Source: CAD feature listing. Evaluate the final solid. Frame: model axes, mm. Round coordinates to 2 decimals unless told otherwise and drop trailing zeros. Loops run counter-clockwise (first coordinate to the right, second up) from the corner with the lowest first, then second, coordinate; pieces in that order, holes last.
Item 1: Section query A-A on z = 23.57. Return loops of the section in (x, y).
Item 2: Section query B-B on x = -42.12. Return loops of the section in (y, z), then the cut area to 3 significant figures.
Item 3: Section query D-D on x = -17.5. Return loops of the section in (y, z).
Item 4: Ray query, L1, parallel to X at y = 1.5, z = -23.57; L2, parallel to Z at x = 32, y = 2.1; L3, parallel to Z at x = -30.5, y = 0.7. Return the intervals inside material, ascending.
Item 5: Section query C-C on x = 32.5. Return loops of the section in (y, z).
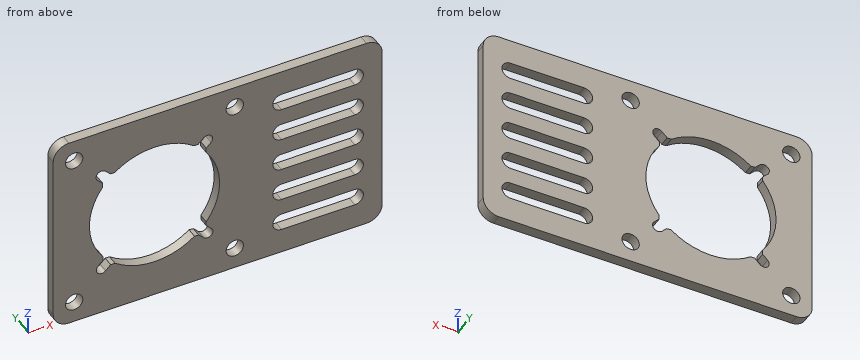
```python
from build123d import *

# Parameters (mm, degrees)
SKETCH1_W           = 96.5
SKETCH1_H           = 60
BOSS_EXTRUDE1_DEPTH = 3
SKETCH2_R           = 2.55
SKETCH2_W           = 26.6
SKETCH2_H           = 5.1
CUT_EXTRUDE1_DEPTH  = 57.895188725
FILLET1_R           = 2.55
FILLET2_R           = 4.6


with BuildPart() as part:
    # Sketch1 → Boss-Extrude1 (new body)
    with BuildSketch(Plane(origin=(0, 0, 0), x_dir=(1, 0, 0), z_dir=(0, 1, 0))):
        Rectangle(SKETCH1_W, SKETCH1_H)
    extrude(amount=BOSS_EXTRUDE1_DEPTH)

    # Sketch2 → Cut-Extrude1 (cut, through all)
    with BuildSketch(Plane(origin=(0, 3, 0), x_dir=(1, 0, 0), z_dir=(0, 1, 0))):
        with Locations(Location((-42.12, 23.57, 0), (0, 0, 270))):
            Circle(SKETCH2_R)
        with Locations(Location((5.02, 23.57, 0), (0, 0, 270))):
            Circle(SKETCH2_R)
        with Locations(Location((5.02, -23.57, 0), (0, 0, 270))):
            Circle(SKETCH2_R)
        with Locations(Location((-42.12, -23.57, 0), (0, 0, 270))):
            Circle(SKETCH2_R)
        with Locations((29.45, 20)):
            Rectangle(SKETCH2_W, SKETCH2_H)
        with Locations((29.45, 10)):
            Rectangle(SKETCH2_W, SKETCH2_H)
        with Locations((29.45, 0)):
            Rectangle(SKETCH2_W, SKETCH2_H)
        with Locations((29.45, -10)):
            Rectangle(SKETCH2_W, SKETCH2_H)
        with Locations((29.45, -20)):
            Rectangle(SKETCH2_W, SKETCH2_H)
        with BuildLine():
            Line((-5.569839705, 15.180766292), (-4.144713605, 16.599616741))
            ThreePointArc((-4.144713605, 16.599616741), (-1.881977414, 16.594623682), (-1.886970473, 14.331887491))
            Line((-1.886970473, 14.331887491), (-3.365955143, 12.859415643))
            Line((-3.365955143, 12.859415643), (-3.36875518, 11.590504981))
            ThreePointArc((-3.36875518, 11.590504981), (0.549812749, -0.084575096), (-3.471995372, -11.72449472))
            Line((-3.471995372, -11.72449472), (-3.369233708, -12.980160295))
            Line((-3.369233708, -12.980160295), (-1.950383259, -14.405286395))
            ThreePointArc((-1.950383259, -14.405286395), (-1.955376318, -16.668022586), (-4.218112509, -16.663029527))
            Line((-4.218112509, -16.663029527), (-5.690584357, -15.184044857))
            Line((-5.690584357, -15.184044857), (-6.959495019, -15.18124482))
            ThreePointArc((-6.959495019, -15.18124482), (-18.634575096, -19.099812749), (-30.27449472, -15.078004628))
            Line((-30.27449472, -15.078004628), (-31.530160295, -15.180766292))
            Line((-31.530160295, -15.180766292), (-32.955286395, -16.599616741))
            ThreePointArc((-32.955286395, -16.599616741), (-35.218022586, -16.594623682), (-35.213029527, -14.331887491))
            Line((-35.213029527, -14.331887491), (-33.734044857, -12.859415643))
            Line((-33.734044857, -12.859415643), (-33.73124482, -11.590504981))
            ThreePointArc((-33.73124482, -11.590504981), (-37.649812749, 0.084575096), (-33.628004628, 11.72449472))
            Line((-33.628004628, 11.72449472), (-33.730766292, 12.980160295))
            Line((-33.730766292, 12.980160295), (-35.149616741, 14.405286395))
            ThreePointArc((-35.149616741, 14.405286395), (-35.144623682, 16.668022586), (-32.881887491, 16.663029527))
            Line((-32.881887491, 16.663029527), (-31.409415643, 15.184044857))
            Line((-31.409415643, 15.184044857), (-30.140504981, 15.18124482))
            ThreePointArc((-30.140504981, 15.18124482), (-18.465424904, 19.099812749), (-6.82550528, 15.078004628))
            Line((-6.82550528, 15.078004628), (-5.569839705, 15.180766292))
        make_face()
    extrude(amount=-CUT_EXTRUDE1_DEPTH, mode=Mode.SUBTRACT)

    # Fillet1
    fillet1_edges = [part.edges().sort_by_distance(p)[0] for p in [
        (42.75, 1.5, 12.55),
        (42.75, 1.5, 22.55),
        (42.75, 1.5, 17.45),
        (42.75, 1.5, 7.45),
        (42.75, 1.5, 2.55),
        (42.75, 1.5, -2.55),
        (42.75, 1.5, -7.45),
        (42.75, 1.5, -12.55),
        (42.75, 1.5, -17.45),
        (42.75, 1.5, -22.55),
        (16.15, 1.5, -17.45),
        (16.15, 1.5, -22.55),
        (16.15, 1.5, 22.55),
        (16.15, 1.5, 17.45),
        (16.15, 1.5, 12.55),
        (16.15, 1.5, 7.45),
        (16.15, 1.5, 2.55),
        (16.15, 1.5, -2.55),
        (16.15, 1.5, -7.45),
        (16.15, 1.5, -12.55),
    ]]
    fillet(fillet1_edges, radius=FILLET1_R - 0.0001)  # a hair under: the kernel refuses the full size

    # Fillet2
    fillet2_edges = [part.edges().sort_by_distance(p)[0] for p in [
        (-48.25, 1.5, -30),
        (48.25, 1.5, -30),
        (48.25, 1.5, 30),
        (-48.25, 1.5, 30),
    ]]
    fillet(fillet2_edges, radius=FILLET2_R)


solid = part.part
```
Data:
1. outline: (-48.25, 0) - (-44.67, 0) - (-44.67, 3) - (-48.25, 3) - close; (-39.57, 0) - (2.47, 0) - (2.47, 3) - (-39.57, 3) - close; (7.57, 0) - (48.25, 0) - (48.25, 3) - (7.57, 3) - close
2. outline: (0, -30) - (3, -30) - (3, -26.12) - (0, -26.12) - close; (0, -21.02) - (3, -21.02) - (3, 21.02) - (0, 21.02) - close; (0, 26.12) - (3, 26.12) - (3, 30) - (0, 30) - close
2. area: 149 mm2
3. outline: (0, -30) - (3, -30) - (3, -19.07) - (0, -19.07) - close; (0, 19.07) - (3, 19.07) - (3, 30) - (0, 30) - close
4. L1: x = -48.25 to -44.67, -39.57 to 2.47, 7.57 to 48.25
4. L2: z = -30 to -22.55, -17.45 to -12.55, -7.45 to -2.55, 2.55 to 7.45, 12.55 to 17.45, 22.55 to 30
4. L3: z = -30 to -15.18, 15.1 to 30
5. outline: (0, -30) - (3, -30) - (3, -22.55) - (0, -22.55) - close; (0, -17.45) - (3, -17.45) - (3, -12.55) - (0, -12.55) - close; (0, -7.45) - (3, -7.45) - (3, -2.55) - (0, -2.55) - close; (0, 2.55) - (3, 2.55) - (3, 7.45) - (0, 7.45) - close; (0, 12.55) - (3, 12.55) - (3, 17.45) - (0, 17.45) - close; (0, 22.55) - (3, 22.55) - (3, 30) - (0, 30) - close
